For this review, take the finished solid that the model builds, in its own axes (mm). A direction names the side the tool comes from. Coordinates: 2 decimals unless noted, no trailing zeros. Order: outer loops, then holes, each group sorted by start corner. A loop starts at its lowest first (then second) coordinate and runs counter-clockwise, first axis right, second up. Notation, with made-up numbers: (-39.5, 20.25) -> (-29.5, 20.25) arc R16 ccw to (-29.5, 47.25) -> close; hole circle Ø9 at (53.5, -39). An arc over 180 degrees is marked (long way). Return JSON: item names as keys, results as strings. Group by question number.
Item 1: Take a section at B-B (z = 130.5). Write out the cut boundary in (x, y).
Item 2: For line 1 along Z through (x, y) = (111, 56.5), list the stretches that pass through material, from the lowest coordinate up.
Item 3: Machinability: for faces 1 (the flat face through (101, 64, 558.8)), 2 (the flat face through (0, 50, 351)), which of the approach directions +Z, -Z, +X, -X, +Y, -Y give a long, thin tool a straight path to every point of the face, cutting with its end or side? Answer none if there is none.
Item 4: Take a section at C-C (x = 112). Write out the cut boundary in (y, z).
Item 5: Draft analysis for pull direction Z (two halves, no side actions). For faces 3 (the flat face through (101, 64, 101.6)), 4 (the flat face through (101, 25.4, 139)), 5 (the flat face through (100, 52, 0)), 6 (the flat face through (203.2, 50, 351)), state which applies: +Z half, -Z half, draft (parallel to the pull), parting line (faces both ways), or undercut.
Item 6: Take a section at A-A (y = 82). Write out the cut boundary in (x, z), then the cut area to 3 significant figures.
```python
from build123d import *

# Parameters (mm, degrees)
SKETCH1_W           = 203.2
SKETCH1_H           = 101.6
BOSS_EXTRUDE1_DEPTH = 711.2
SKETCH2_W           = 76.2
SKETCH2_H           = 76.2
CUT_EXTRUDE1_DEPTH  = 76.2


with BuildPart() as part:
    # Sketch1 → Boss-Extrude1 (new body)
    with BuildSketch(Plane.XY):
        with Locations((101.6, 50.8)):
            Rectangle(SKETCH1_W, SKETCH1_H)
    extrude(amount=BOSS_EXTRUDE1_DEPTH)

    # Sketch2 → Cut-Extrude1 (cut)
    with BuildSketch(Plane(origin=(0, 101.6, 0), x_dir=(1, 0, 0), z_dir=(0, 1, 0))):
        with Locations((101.6, -139.7)):
            Rectangle(SKETCH2_W, SKETCH2_H)
        with Locations((101.6, -596.9)):
            Rectangle(SKETCH2_W, SKETCH2_H)
    extrude(amount=-CUT_EXTRUDE1_DEPTH, mode=Mode.SUBTRACT)


solid = part.part
```
Findings below:
{
 "1": {"outline": "(0, 0) -> (203.2, 0) -> (203.2, 101.6) -> (139.7, 101.6) -> (139.7, 25.4) -> (63.5, 25.4) -> (63.5, 101.6) -> (0, 101.6) -> close"},
 "2": {"line 1": "z = 0 to 101.6, 177.8 to 558.8, 635 to 711.2"},
 "3": {"face 1": "+Y", "face 2": "+Z, -Z, -X, +Y, -Y"},
 "4": {"outline": "(0, 0) -> (101.6, 0) -> (101.6, 101.6) -> (25.4, 101.6) -> (25.4, 177.8) -> (101.6, 177.8) -> (101.6, 558.8) -> (25.4, 558.8) -> (25.4, 635) -> (101.6, 635) -> (101.6, 711.2) -> (0, 711.2) -> close"},
 "5": {"face 3": "undercut", "face 4": "undercut", "face 5": "-Z half", "face 6": "draft"},
 "6": {"outline": "(0, 0) -> (203.2, 0) -> (203.2, 711.2) -> (0, 711.2) -> close; hole (63.5, 101.6) -> (139.7, 101.6) -> (139.7, 177.8) -> (63.5, 177.8) -> close; hole (63.5, 558.8) -> (139.7, 558.8) -> (139.7, 635) -> (63.5, 635) -> close", "area": "133,000 mm2"}
}
